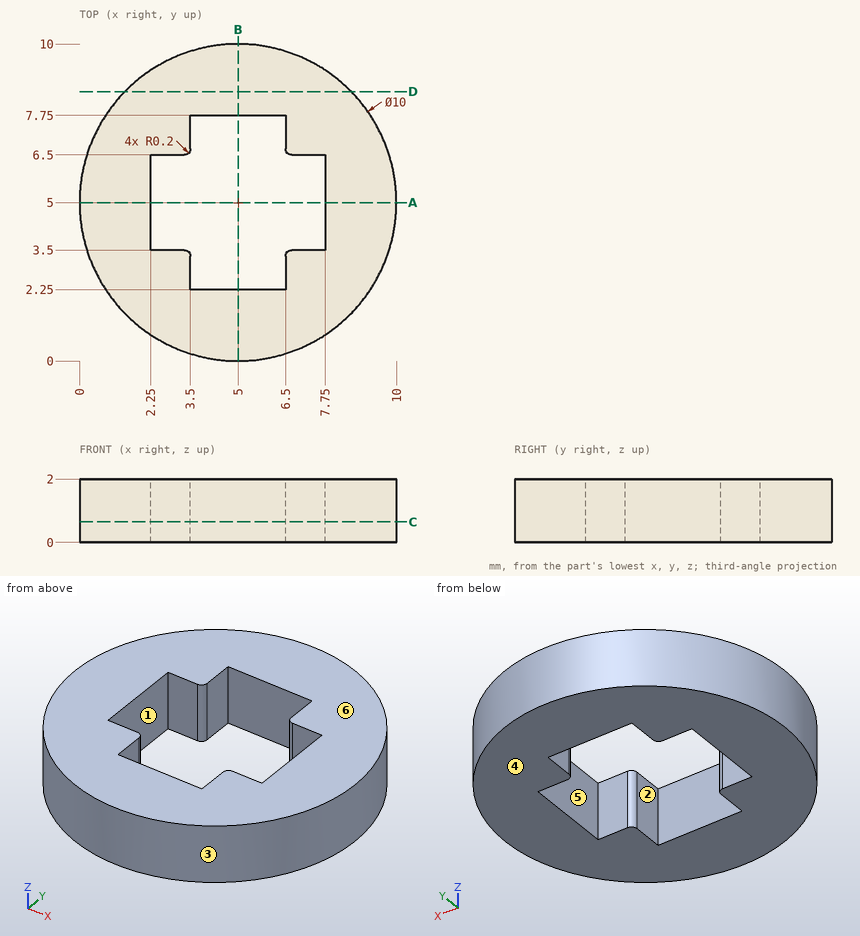
Study the drawing (mm; zero at the part's minimum x, y, z) and answer. A direction names the side the tool comes from. Give positions to 0.01 mm unless a question says otherwise; leave off trailing zeros. Write each loop counter-clockwise with the first axis right and the second up, starting at its lowest first coordinate (ties: lowest second). Pieces come first, ordered by that corner, then holes.
Item 1: Section C-C, the plane z = 0.65 is taken. Write down the section's boundary in (x, y), plus the area to 3 significant figures.
Item 2: Section D-D, the plane y = 8.5 is taken. Write down the section's boundary in (x, z), plus the area to 3 significant figures.
Item 3: Which of the six approach directions +Z, -Z, +X, -X, +Y, -Y give full straight-line access (tool end or side, diameter ignored) to the marked faces 5 and 6?
Item 4: Find the intervals of material crossed by line 1 along Y through (x, z) = (6.75, 1.9); line 2 along Y through (x, z) = (5.25, 1.15); line 3 along X through (y, z) = (2.75, 1.2), in increasing order.
Item 5: Flat-ended cylindrical pins translate along their axes: P1, Ø0.8, axis at x = 3, z = 1, coming from the -Y side; P2, Ø0.6, axis at x = 4.5, z = 1, coming from the -Y side; P3, Ø0.6, axis at y = 5.5, z = 1, coming from the -X side. Find the tip coordinate at first contact, or state that the pin passes through.
Item 6: Section A-A, the plane y = 5 is taken. Write down the section's boundary in (x, z), plus the area to 3 significant figures.
Item 7: Determine the mould class of the marked faces 1, 2, 3 and 4 for opening direction Y: released by +Y, released by -Y, zero draft, split by the parting line, or undercut.
Completed:
1. outline: circle Ø10 at (5, 5); hole (2.25, 3.5) - (3.3, 3.5) arc R0.2 cw to (3.5, 3.3) - (3.5, 2.25) - (6.5, 2.25) - (6.5, 3.3) arc R0.2 cw to (6.7, 3.5) - (7.75, 3.5) - (7.75, 6.5) - (6.7, 6.5) arc R0.2 cw to (6.5, 6.7) - (6.5, 7.75) - (3.5, 7.75) - (3.5, 6.7) arc R0.2 cw to (3.3, 6.5) - (2.25, 6.5) - close
1. area: 54.5 mm2
2. outline: (1.43, 0) - (8.57, 0) - (8.57, 2) - (1.43, 2) - close
2. area: 14.3 mm2
3. face 5: +Z, -Z
3. face 6: +Z, +X, -X, +Y, -Y
4. line 1: y = 0.32 to 3.5, 6.5 to 9.68
4. line 2: y = 0.01 to 2.25, 7.75 to 9.99
4. line 3: x = 0.53 to 3.5, 6.5 to 9.47
5. P1: stops at y = 0.26
5. P2: stops at y = 0
5. P3: stops at x = 0
6. outline: (0, 0) - (2.25, 0) - (2.25, 2) - (0, 2) - close; (7.75, 0) - (10, 0) - (10, 2) - (7.75, 2) - close
6. area: 9.00 mm2
7. face 1: undercut
7. face 2: undercut
7. face 3: split by the parting line
7. face 4: zero draft
